Geometry check sheet. Reference: the model listing, model coordinates, mm. A direction names the side the tool comes from. Round coordinates to 2 decimals unless told otherwise and drop trailing zeros. Loops run counter-clockwise (first coordinate to the right, second up) from the corner with the lowest first, then second, coordinate; pieces in that order, holes last.
```python
from build123d import *

# Parameters (mm, degrees)
F0_R      = 78.74
F0_R_2    = 63.5
F1_DEPTH  = 50.8
F2_R      = 63.5
F2_R_2    = 52.07
F5_DEPTH  = 48.26
F4_R      = 63.5
F4_R_2    = 40.64
F6_DEPTH  = 38.1
F3_W      = 5.037099
F3_H      = 46.096297
F8_W      = 9.554964
F8_H      = 33.442384
F10_R     = 15.24
F11_DEPTH = 70.999706


with BuildPart() as f1:
    # F0 (on Front) → F1 (new body)
    with BuildSketch(Plane.XZ):
        Circle(F0_R)
        Circle(F0_R_2, mode=Mode.SUBTRACT)
    extrude(amount=F1_DEPTH)

    # F2 (on Front) → F5 (join)
    with BuildSketch(Plane.XZ):
        Circle(F2_R)
        Circle(F2_R_2, mode=Mode.SUBTRACT)
    extrude(amount=F5_DEPTH)

    # F4 (on Front) → F6 (join)
    with BuildSketch(Plane.XZ):
        Circle(F4_R)
        Circle(F4_R_2, mode=Mode.SUBTRACT)
    extrude(amount=F6_DEPTH)

    # F3 (on Right) → F7 (revolve)
    with BuildSketch(Plane.YZ):
        Polygon((42.333808, 78.692965), (24.474939, 78.692965), (24.474939, 1.865802), (42.333808, 1.865802), (42.333808, 52.154191), align=None)
        with BuildLine():
            Line((24.474939, 1.865802), (24.474939, 78.692965))
            ThreePointArc((24.474939, 78.692965), (12.23747, 66.455496), (0, 78.692965))
            Line((0, 78.692965), (0, 1.865802))
            Line((0, 1.865802), (24.474939, 1.865802))
        make_face()
        Polygon((65.961607, 52.154191), (42.333808, 52.154191), (42.333808, 1.865802), (65.961607, 1.865802), (65.961607, 47.962099), align=None)
        with Locations((68.480156, 24.91395)):
            Rectangle(F3_W, F3_H)
    revolve(axis=Axis((0, 23.528613, 0), (0, 1, 0)))

    # F8 (on Right) → F9 (revolve, cut)
    with BuildSketch(Plane.YZ):
        Polygon((-29.593855, 39.679654), (-29.593855, 6.23727), (-21.365967, 6.23727), (-21.365967, 50.296281), (-29.593855, 50.296281), align=None)
        with Locations((-34.371337, 22.958462)):
            Rectangle(F8_W, F8_H)
    revolve(axis=Axis((0, -25.413556, 0), (0, -1, 0)), mode=Mode.SUBTRACT)

    # F10 (on Front) → F11 (cut, through all)
    with BuildSketch(Plane.XZ):
        Circle(F10_R)
    extrude(amount=-F11_DEPTH, mode=Mode.SUBTRACT)


solid = f1.part
```
1) Gauge pin test, flat ends, axial feed: pin 1 (12 mm diameter, centred on x = 41, z = -43, fed in from +Y); pin 2 (1 mm diameter, centred on x = 57.5, y = -32.5, fed in from -Z); pin 3 (10 mm diameter, centred on x = -30.5, y = 14.5, fed in from -Z). Record the tip position at first contact, or that the pin passes through.
Report:
pin 1: stops at y = 42.33
pin 2: stops at z = -54.32
pin 3: stops at z = -62.39
2) Sectioned sample at B-B, the plane y = 59.5. Record the cut outline in (x, z).
Report:
outline: circle Ø104.31 at (0, 0); hole circle Ø30.48 at (0, 0)
3) Scan lines: line 1 along Z through (x, y) = (0, -48.9); line 2 along Z through (x, y) = (0, -27); line 3 along Y through (x, z) = (-28, -66.5). Record each from-to range of solid material in increasing order.
Report:
line 1: z = -78.74 to -63.5, 63.5 to 78.74
line 2: z = -78.74 to -50.3, 50.3 to 78.74
line 3: y = -50.8 to 1.89, 22.58 to 42.33
4) Access from +Z, -Z, +X, -X, +Y, -Y to the whole of each face (thin tool, end or side, straight path). Record for faces 1 (the face through (-29.184, 68.515, -38.061)), 2 (the face through (-13.77, -49.51, -61.99)), 3 (the face through (0, -21.366, -41)).
Report:
face 1: +Y
face 2: -Y
face 3: none
5) Sectioned sample at A-A, the plane y = -26. Record the cut outline in (x, z), then the cut area to 3 significant figures.
Report:
outline: circle Ø157.48 at (0, 0); hole circle Ø100.59 at (0, 0)
area: 11,500 mm2
6) Mould release check, pull along X, two halves, no side actions. Record for faces 4 (the face through (11, 70.999, 11)), 5 (the face through (-5, -48.26, 52)), 6 (the face through (15.666, 53.982, 49.746)): +X half, -X half, draft (parallel to the pull), parting line (faces both ways), or undercut.
Report:
face 4: draft
face 5: undercut
face 6: parting line
